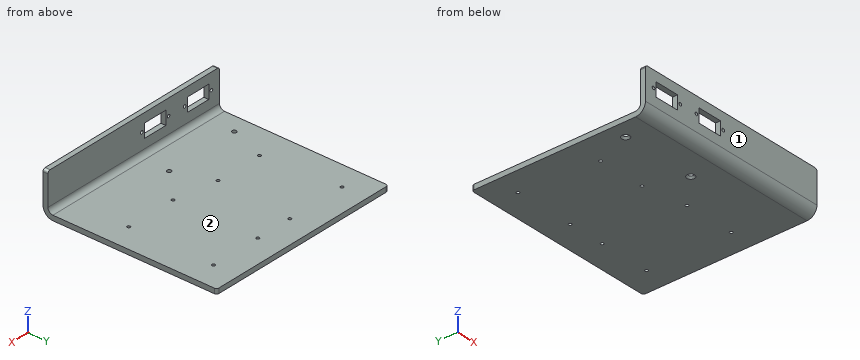
Autodesk Inventor part; units mm, degrees
ref_plane "Plan YZ" through (0, 0, 0) normal (1, 0, 0) x (0, 1, 0)
ref_plane "Plan XZ" through (0, 0, 0) normal (0, 1, 0) x (-1, 0, 0)
ref_plane "Plan XY" through (0, 0, 0) normal (0, 0, 1) x (1, 0, 0)
sketch "Esquisse1" plane through (0, 0, 0) normal (0, 0, 1) x (1, 0, 0)
  line L0 (-78, 70) -> (78, 70)
  line L1 (80, 68) -> (80, -68)
  line L2 (78, -70) -> (-78, -70)
  line L3 (-80, -68) -> (-80, 68)
  line L4 (-112, 0) -> (112, 0) construction
  line L5 (0, -98) -> (0, 98) construction
  line L6 (-80, 68) -> (-80, 70)
  line L7 (-80, 70) -> (-78, 70)
  line L8 (80, 68) -> (80, 70)
  line L9 (78, 70) -> (80, 70)
  line L10 (-78, -70) -> (-80, -70)
  line L11 (-80, -70) -> (-80, -68)
  line L12 (78, -70) -> (80, -70)
  line L13 (80, -70) -> (80, -68)
  point P0 (0, 0)
  dimension "d0" = 160
  dimension "d1" = 140
extrude "Extrusion1" add sketch "Esquisse1" along normal blind 4
sketch "Esquisse5" plane through (0, 0, 4) normal (0, 0, 1) x (1, 0, 0)
  line L0 (18.6, 50) -> (60, 50) construction
  line L1 (60, 50) -> (60, -18.2) construction
  line L2 (60, -18.2) -> (18.6, -18.2) construction
  line L3 (18.6, -18.2) -> (18.6, 50) construction
  line L4 (80, -70.465) -> (80, 70)
  line L5 (80, 70) -> (-80, 70)
  line L6 (80, 70) -> (-80, 70)
  line L7 (80, -70) -> (80, 70)
  point P0 (0, 0)
  point P1 (0, 0)
  point P2 (78, 70)
  point P3 (-78, 70)
  point P4 (80, -68)
  point P5 (80, 68)
  dimension "d12" = 41.4
  dimension "d13" = 68.2
  dimension "d14" = 20
  dimension "d15" = 20
hole "Perçage1" at (18.6, 50, 4) at (60, 50, 4) at (18.6, -18.2, 4) at (60, -18.2, 4) direction (0, 0, -1) diameter 2.459 end through all
sketch "Esquisse6" plane through (0, 0, 4) normal (0, 0, 1) x (1, 0, 0)
  line L0 (-60, 50) -> (-11.3, 50) construction
  line L1 (-11.3, 50) -> (-11.3, -12.2) construction
  line L2 (-11.3, -12.2) -> (-60, -12.2) construction
  line L3 (-60, -12.2) -> (-60, 50) construction
  line L4 (-35.65, 66.5768) -> (-35.65, 16.8329)
  line L5 (-80, 70) -> (-80, -63.3699)
  line L6 (-80, 70) -> (-80, -70) construction
  line L7 (80, 70) -> (-80, 70)
  circle A0 centre (18.6, 50) radius 1.2295 construction
  point P0 (0, 0)
  point P1 (0, 0)
  point P2 (-54.9, -12.2)
  point P3 (-16.4, -12.2)
  point P4 (-80, 68)
  point P5 (-80, -68)
  point P6 (78, 70)
  point P7 (-78, 70)
  dimension "d23" = 62.2
  dimension "d24" = 38.5
  dimension "d25" = 48.7
  dimension "d26" = 48.7
  dimension "d27" = 20
hole "Perçage2" at (-54.9, -12.2, 4) at (-16.4, -12.2, 4) at (-60, 50, 4) at (-11.3, 50, 4) direction (0, 0, -1) diameter 2.459 end through all
sketch "Esquisse10" plane through (80, -66, 0) normal (0, -1, 0) x (1, 0, 0)
  line L0 (-160, 0) -> (0, 0)
  line L1 (0, 0) -> (0, 34)
  line L2 (0, 34) -> (-160, 34)
  line L3 (-160, 34) -> (-160, 0)
edge flange "Bord tombé2" height 34 angle 90 thickness 4 bend radius 4 thickness toward (0, -1, 0) relief straight relief width 4 relief depth 2 edges at (0, -70, 4) wall of the first edge with corners at (-80, -66, 0) (80, -66, 0) (80, -66, 34) (-80, -66, 34)
bend "Pli3"
corner "Coin2"
fillet "Congé1" radius 2 4 edges at (-80, -68, 34) (80, -68, 34) (80, 70, 2) (-80, 70, 2)
sketch "Esquisse13" plane through (0, 0, 0) normal (0, 0, -1) x (-1, 0, 0)
  line L0 (35.65, 25.8994) -> (35.65, -17.0856) construction
  line L1 (80, -70) -> (-80, -70) construction
  line L2 (80, 70) -> (80, -62) construction
  line L3 (151.9558, 0) -> (-118.6593, 0) construction
  line L4 (80, -62) -> (-80, -62)
  point P0 (0, 0)
  point P1 (0, 0)
  point P2 (0, 0)
  point P3 (66.05, -42)
  point P4 (5.25, -42)
  point P5 (16.4, 8.1)
  point P6 (80, 68)
  dimension "d102" = 38.5
  dimension "d107" = 60.8
  dimension "d115" = 20
hole "Perçage4" at (-5.25, -42, 0) at (-66.05, -42, 0) direction (0, 0, 1) diameter 3.4 end through all countersink diameter 6.3 countersink angle 90
sketch "Esquisse12" plane through (-80, -70, 8) normal (0, -1, 0) x (1, 0, 0)
  line L0 (10, 18.5) -> (30, 18.5)
  line L1 (30, 18.5) -> (30, 7.5)
  line L2 (30, 7.5) -> (10, 7.5)
  line L3 (10, 7.5) -> (10, 18.5)
  line L4 (50, 18.5) -> (70, 18.5)
  line L5 (70, 18.5) -> (70, 7.5)
  line L6 (70, 7.5) -> (50, 7.5)
  line L7 (50, 7.5) -> (50, 18.5)
  line L8 (2, 26) -> (158, 26)
  line L9 (-10.9148, 13) -> (171.3992, 13)
  line L10 (20, 22.4004) -> (20, 5.8983)
  line L11 (60, 25.3782) -> (60, 6.6427)
  line L12 (0, -0.9203) -> (0, 29.0797)
  line L13 (40, 26) -> (40, -5.9495)
  line L14 (0, 0) -> (0, 26)
  line L15 (0, 26) -> (160, 26)
  point P0 (80, -8)
  point P1 (80, -2)
  point P2 (0, 24)
  point P3 (2, 26)
  point P4 (158, 26)
  point P5 (7.503, 13)
  point P6 (32.497, 13)
  point P7 (47.503, 13)
  point P8 (72.497, 13)
  dimension "d81" = 26
  dimension "d82" = 11
  dimension "d83" = 20
  dimension "d84" = 20
  dimension "d85" = 20
  dimension "d89" = 20
  dimension "d90" = 80
  dimension "d116" = 24.994
  dimension "d117" = 24.994
extrude "Extrusion5" cut sketch "Esquisse12" against normal through all contours L0 L10 L9 L3 | L0 L1 L9 L10 | L9 L10 L2 L3 | L9 L1 L2 L10 | L4 L11 L9 L7 | L4 L5 L9 L11 | L9 L11 L6 L7 | L9 L5 L6 L11
hole "Perçage5" at (-72.497, -70, 21) at (-47.503, -70, 21) at (-32.497, -70, 21) at (-7.503, -70, 21) direction (0, 1, 0) diameter 2.459 end through all
equation "\"d26\" = d25"
equation "\"d113\" = Epaisseur"
equation "\"d90\" = 0.5 * d91"
equation "\"d65\" = LargeurGrugeage"
equation "\"d66\" = ProfondeurGrugeage"
equation "\"d67\" = RestesMinimum"
equation "\"d68\" = RayonPli"
equation "\"d71\" = RayonPli"
equation "\"d72\" = TailleGrugeage"
equation "\"d73\" = TailleJeu"
equation "\"d74\" = TailleRayonJacobi"
equation "\"RayonPli\" = Epaisseur"
equation "\"LargeurGrugeage\" = Epaisseur"
equation "\"ProfondeurGrugeage\" = 0.5 * Epaisseur"
equation "\"TailleGrugeage\" = 4 * Epaisseur"
equation "\"RestesMinimum\" = 2 * Epaisseur"
equation "\"Rayondetransition\" = RayonPli"
equation "\"TailleRayonJacobi\" = Epaisseur"
equation "\"TailleJeu\" = Epaisseur"
properties part number "P1704_007" material "Plastique PMMA"
Geometry: final body of the model. Coordinates: model frame, mm. Face numbers are marked on the shaded views. A direction names the side the tool comes from. Round coordinates to 2 decimals unless told otherwise and drop trailing zeros. Order: outer loops, then holes, each group sorted by start corner. A loop starts at its lowest first (then second) coordinate and runs counter-clockwise, first axis right, second up. Notation, with made-up numbers: (-36.5, -11.5) -> (0.5, -11.5) arc R11 cw to (0.5, 4.5) -> close; hole circle Ø7 at (28.25, -27.5). An arc over 180 degrees is marked (long way). Use one line per item in the form item = value. Start each with the question number.
1. Cut plane A-A (z = 24). Return the cut outline in (x, y), then the cut area to 3 significant figures.
2. Reachability of the marked faces 1 and 2 from +Z, -Z, +X, -X, +Y, -Y: full face, straight path, thin tool, end or side. Return the list, or none.
3. Pin query (flat end, axial travel): pin 1 Ø5 at (x, z) = (53, 23) entering from +Y; pin 2 Ø2 at (x, y) = (-55.5, -68.5) entering from -Z; pin 3 Ø2 at (x, y) = (2.5, -54.5) entering from +Z. Return the tip coordinate at first contact, or that it passes through.
4. Line query: probe 1 along X at (y, z) = (-42, 2); probe 2 along X at (y, z) = (50, 1); probe 3 along X at (y, z) = (-12, 1). Output: solid intervals per line, ascending.
5. Cut plane B-B (y = 6). Return the cut outline in (x, z).
Solution:
q1.outline = (-80, -70) -> (-70, -70) -> (-70, -66) -> (-80, -66) -> close; (-50, -70) -> (-30, -70) -> (-30, -66) -> (-50, -66) -> close; (-10, -70) -> (80, -70) -> (80, -66) -> (-10, -66) -> close
q1.area = 480 mm^2
q2.face_1 = +Z, -Z, +X, -X, -Y
q2.face_2 = +Z, +X, -X, +Y
q3.pin_1 = -66
q3.pin_2 = 2.19
q3.pin_3 = 4
q4.probe_1 = -80 to -67.75, -64.35 to -6.95, -3.55 to 80
q4.probe_2 = -80 to -61.23, -58.77 to -12.53, -10.07 to 17.37, 19.83 to 58.77, 61.23 to 80
q4.probe_3 = -80 to -56.11, -53.69 to -17.61, -15.19 to 80
q5.outline = (-80, 0) -> (80, 0) -> (80, 4) -> (-80, 4) -> close
